```python
from build123d import *

# Parameters (mm, degrees)
F0_W      = 120
F0_H      = 39.79
F1_DEPTH  = 80
F2_W      = 18.18
F2_H      = 18.4
F3_DEPTH  = 30.03
F4_W      = 23
F4_H      = 20.8
F5_DEPTH  = 10.8
F7_DEPTH  = 19.23
F8_R      = 2
F10_DEPTH = 8.25
F12_DEPTH = 120.001
F13_R     = 3
F14_DEPTH = 80.001
F15_R     = 5.5
F15_R_2   = 3
F16_DEPTH = 6


with BuildPart() as f1:
    # F0 (on Front) → F1 (new body)
    with BuildSketch(Plane.XZ):
        with Locations((0, -19.895)):
            Rectangle(F0_W, F0_H)
    extrude(amount=F1_DEPTH)

    # F2 (on face) → F3 (cut)
    with BuildSketch(Plane.XZ.offset(80)):
        with Locations((0, -30.59)):
            Rectangle(F2_W, F2_H)
    extrude(amount=-F3_DEPTH, mode=Mode.SUBTRACT)

    # F4 (on face) → F5 (cut)
    with BuildSketch(Plane.XZ.offset(80)):
        with Locations((0, -29.39)):
            Rectangle(F4_W, F4_H)
    extrude(amount=-F5_DEPTH, mode=Mode.SUBTRACT)

    # F6 (on face) → F7 (cut, through all)
    with BuildSketch(Plane.XZ.offset(69.2)):
        with BuildLine():
            ThreePointArc((-8.59, -20.89), (-9.297107, -21.182893), (-9.59, -21.89))
            ThreePointArc((-9.59, -21.89), (-8.59, -22.89), (-7.59, -21.89))
            ThreePointArc((-7.59, -21.89), (-7.882893, -21.182893), (-8.59, -20.89))
        make_face()
        with BuildLine():
            ThreePointArc((9.59, -21.89), (9.297107, -21.182893), (8.59, -20.89))
            ThreePointArc((8.59, -20.89), (7.882893, -22.597107), (9.59, -21.89))
        make_face()
    extrude(amount=-F7_DEPTH, mode=Mode.SUBTRACT)

    # F8
    f8_edges = [f1.edges().sort_by_distance(p)[0] for p in [
        (-11.5, -74.6, -18.99),
        (11.5, -74.6, -18.99),
    ]]
    fillet(f8_edges, radius=F8_R)

    # F9 (on face) → F10 (cut)
    with BuildSketch(Plane.XZ.offset(80)):
        Polygon((0.2, 0), (-48.998643, 0), (-10.033396, -39.79), (0.2, -39.79), align=None)
        Polygon((49.916624, 0), (0.2, 0), (0.2, -39.79), (10.541137, -39.79), align=None)
    extrude(amount=-F10_DEPTH, mode=Mode.SUBTRACT)

    # F11 (on face) → F12 (cut, through all)
    with BuildSketch(Plane.YZ.offset(60)):
        Polygon((-49, -8.39), (0, -8.39), (0, 0), (-80, 0), (-80, -16.39), (-49, -16.39), align=None)
    extrude(amount=-F12_DEPTH, mode=Mode.SUBTRACT)

    # F13 (on face) → F14 (cut, through all)
    with BuildSketch(Plane(origin=(0, 0, 0), x_dir=(-1, 0, 0), z_dir=(0, 1, 0))):
        with Locations((-53, -28.29)):
            Circle(F13_R)
        with Locations((-36, -28.29)):
            Circle(F13_R)
        with Locations((36, -28.29)):
            Circle(F13_R)
        with Locations((53, -28.29)):
            Circle(F13_R)
    extrude(amount=-F14_DEPTH, mode=Mode.SUBTRACT)

    # F15 (on face) → F16 (cut)
    with BuildSketch(Plane(origin=(0, 0, 0), x_dir=(-1, 0, 0), z_dir=(0, 1, 0))):
        with Locations((-53, -28.29)):
            Circle(F15_R)
        with Locations((-53, -28.29)):
            Circle(F15_R_2, mode=Mode.SUBTRACT)
        with Locations((-36, -28.29)):
            Circle(F15_R)
        with Locations((-36, -28.29)):
            Circle(F15_R_2, mode=Mode.SUBTRACT)
        with Locations((36, -28.29)):
            Circle(F15_R)
        with Locations((36, -28.29)):
            Circle(F15_R_2, mode=Mode.SUBTRACT)
        with Locations((53, -28.29)):
            Circle(F15_R)
        with Locations((53, -28.29)):
            Circle(F15_R_2, mode=Mode.SUBTRACT)
    extrude(amount=-F16_DEPTH, mode=Mode.SUBTRACT)


solid = f1.part
```
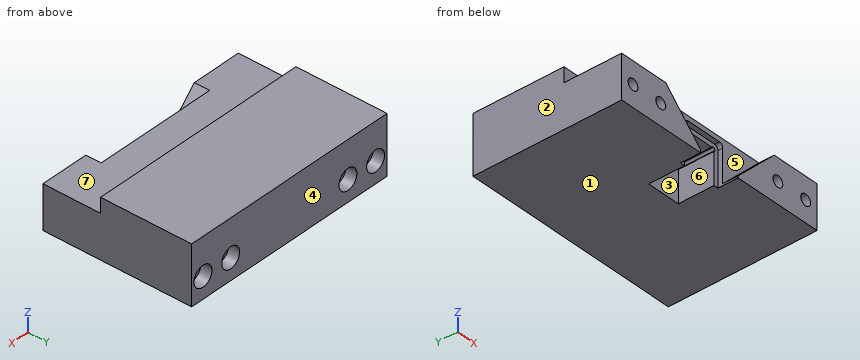
Check sheet for the modelled part. Datum: model origin and axes. Units: mm. Face numbers are marked on the shaded views. A direction names the side the tool comes from. Give positions to 0.01 mm unless a question says otherwise; leave off trailing zeros. Order: outer loops, then holes, each group sorted by start corner. A loop starts at its lowest first (then second) coordinate and runs counter-clockwise, first axis right, second up. Notation, with made-up numbers: M 36.5,47 L 82.5,47 A22 cw 82.5,66 Z; hole C -15,4.25 d5. An arc over 180 degrees is marked long. Answer in a Markdown table with one row per item. Add a question column.
Q1. Sectioned sample at B-B, the plane y = -42. Record the boundary of the cut face in (x, z).
Q2. Sectioned sample at A-A, the plane x = 53. Record the boundary of the cut face in (y, z), and give its area (3 significant figures).
Q3. Access from +Z, -Z, +X, -X, +Y, -Y to the whole of each face (thin tool, end or side, straight path). Record for the marked faces 4, 5, 6 and 7.
Q4. Release check for a two-part mould opening along X. For the marked faces 1, 2 and 3 record: released by +X, released by -X, zero draft, split by the parting line, or undercut.
Q5. Sectioned sample at D-D, the plane z = -28.29. Count the separate pieces of the cut face and the enclosed holes in it, and give its area (3 significant figures).
Q6. Gauge pin test, flat ends, axial feed: pin 1 Ø5.5 at (x, z) = (51, -28.5) entering from +Y; pin 2 Ø4.5 at (x, y) = (2, -61.5) entering from -Z; pin 3 Ø5.5 at (x, z) = (-2.5, -26.5) entering from -Y. Record the tip position at first contact, or that the pin passes through.
Q7. Thickness scan on L1, parallel to X at y = -1, z = -28; L2, parallel to Z at x = -53, y = -1.8; L3, parallel to Z at x = 36, y = -45. Record the ranges inside material, lowest first.
Q8. Sectioned sample at C-C, the plane x = 4. Record the boundary of the cut face in (y, z).
Verdict:
| question | item | result |
|---|---|---|
| 1 | outline | M -60,-39.79 L 60,-39.79 L 60,-8.39 L -60,-8.39 Z; hole C -53,-28.29 d6; hole C -36,-28.29 d6; hole C 36,-28.29 d6; hole C 53,-28.29 d6 |
| 2 | outline | M -80,-39.79 L 0,-39.79 L 0,-33.79 L -6,-33.79 L -6,-31.29 L -80,-31.29 Z; M -80,-25.29 L -6,-25.29 L -6,-22.79 L 0,-22.79 L 0,-8.39 L -49,-8.39 L -49,-16.39 L -80,-16.39 Z |
| 2 | area | 1,750 mm² |
| 3 | face 4 | +Z, -Z, +X, -X, +Y |
| 3 | face 5 | +Z, -Y |
| 3 | face 6 | -Z, -Y |
| 3 | face 7 | +Z, +X, -X, -Y |
| 4 | face 1 | zero draft |
| 4 | face 2 | released by -X |
| 4 | face 3 | undercut |
| 5 | separate pieces | 5 |
| 5 | enclosed holes | 0 |
| 5 | area | 6,800 mm² |
| 6 | pin 1 | y = -6 |
| 6 | pin 2 | z = -21.39 |
| 6 | pin 3 | y = -49.97 |
| 7 | L1 | -60 to -58.49, -47.51 to -41.49, -30.51 to 30.51, 41.49 to 47.51, 58.49 to 60 |
| 7 | L2 | -39.79 to -33.79, -22.79 to -8.39 |
| 7 | L3 | -39.79 to -31.29, -25.29 to -8.39 |
| 8 | outline | M -71.75,-18.99 L -69.2,-18.99 L -69.2,-21.39 L -49.97,-21.39 L -49.97,-39.79 L 0,-39.79 L 0,-8.39 L -49,-8.39 L -49,-16.39 L -71.75,-16.39 Z |
